```python
from build123d import *


with BuildPart() as part:
    # Skizze1 → Rotation1 (revolve)
    with BuildSketch(Plane.XY, mode=Mode.PRIVATE) as rotation1_sk:
        with BuildLine():
            Line((0, 0), (13.150358125, 2))
            ThreePointArc((13.150358125, 2), (13.997153849, 3.064025241), (13, 3.988631597))
            Line((13, 3.988631597), (13, 6.998384988))
            ThreePointArc((13, 6.998384988), (14, 7.998384988), (13, 8.998384988))
            Line((13, 8.998384988), (8.5, 8.998384988))
            Line((8.5, 8.998384988), (8.5, 5.998384988))
            Line((8.5, 5.998384988), (10.5, 5.998384988))
            Line((10.5, 5.998384988), (10.5, 2.998384988))
            Line((10.5, 2.998384988), (0, 2.998384988))
            Line((0, 2.998384988), (0, 0))
        make_face()
    revolve(rotation1_sk.sketch.rotate(Axis((0, 0, 0), (0, 1, 0)), 90), axis=Axis((0, 0, 0), (0, 1, 0)))


solid = part.part
```
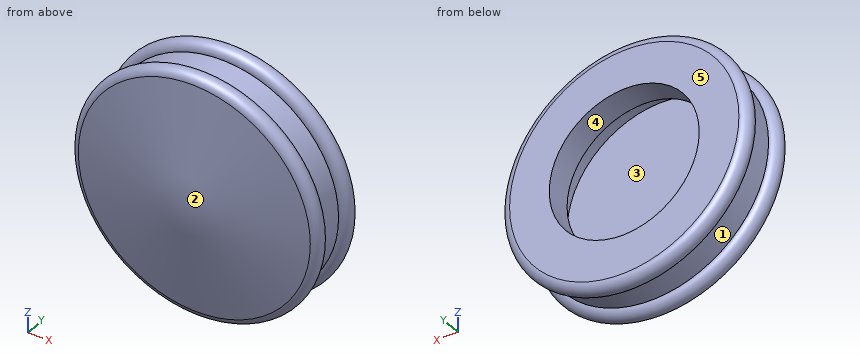
Verification items for the finished model (mm, model axes). Face numbers are marked on the shaded views. A direction names the side the tool comes from. Coordinates: 2 decimals unless noted, no trailing zeros. Order: outer loops, then holes, each group sorted by start corner. A loop starts at its lowest first (then second) coordinate and runs counter-clockwise, first axis right, second up. Notation, with made-up numbers: (75.5, 13.5) -> (118.5, 13.5) arc R8 cw to (118.5, 27.5) -> close; hole circle Ø3 at (22.25, 45.25). An arc over 180 degrees is marked (long way). Put each result on its own line as item: value. Start each with the question number.
1) Cross-section at B-B (y = 0.5). Enter the section's corners in (x, z).
2) Tool access check on the marked faces 1 and 2. Record the directions out of +Z, -Z, +X, -X, +Y, -Y that give a thin tool (end or side, any length) a straight path to the whole face; none if there is none.
3) Cross-section at A-A (y = 4.5). Enter the section's corners in (x, z), plus the area to 3 significant figures.
4) Material ranges on L1, parallel to X at y = 4.4, z = 0; L2, parallel to X at y = 6.5, z = -5.75; L3, parallel to Y at x = -2.75, z = -8.5, recorded low to high.
5) Go/stop test with flat-tipped pins: pin 1 (6.5 mm diameter, centred on x = 4, z = 0, fed in from +Y); pin 2 (3 mm diameter, centred on y = 2, z = -2, fed in from -X); pin 3 (5 mm diameter, centred on y = 4, z = -3, fed in from +X). Record where each tip stops, or that it passes through.
6) Release check for a two-part mould opening along Y. For the marked faces 3, 4 and 5 record: pulls with the +Y half, pulls with the -Y half, needs draft (parallel to the pull), parting line crosses it, or undercut.
Geometry check:
1. outline: circle Ø6.58 at (0, 0)
2. face 1: none
2. face 2: -Y
3. outline: circle Ø26 at (0, 0); hole circle Ø21 at (0, 0)
3. area: 185 mm^2
4. L1: x = -13 to -10.5, 10.5 to 13
4. L2: x = -11.66 to -6.26, 6.26 to 11.66
4. L3: y = 1.36 to 3, 6 to 9
5. pin 1: stops at y = 3
5. pin 2: stops at x = -13.97
5. pin 3: stops at x = 13.98
6. face 3: undercut
6. face 4: needs draft
6. face 5: pulls with the +Y half
